Input: part model. Units: mm. Frame: model coordinates. Round coordinates to 2 decimals unless told otherwise and drop trailing zeros. Order: outer loops, then holes, each group sorted by start corner. A loop starts at its lowest first (then second) coordinate and runs counter-clockwise, first axis right, second up. Notation, with made-up numbers: (83.25, -27) -> (97.25, -27) arc R24 cw to (97.25, 4) -> close; hole circle Ø3 at (29.25, -19.5). An arc over 180 degrees is marked (long way). Use a Markdown table: item, result.
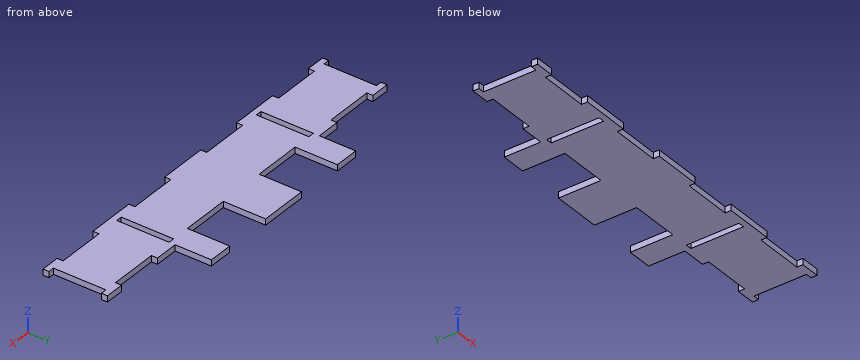
from build123d import *

# Parameters (mm, degrees)
SKETCH1_W           = 395.4
SKETCH1_H           = 67.700000012
BOSS_EXTRUDE1_DEPTH = 6.35
SKETCH2_W           = 50.8
SKETCH2_H           = 6.35
SKETCH2_W_2         = 6.35
SKETCH2_H_2         = 55.000000012
CUT_EXTRUDE1_DEPTH  = 201.677440188
SKETCH5_W           = 6.35
SKETCH5_H           = 55.000000012
CUT_EXTRUDE2_DEPTH  = 201.677440188
SKETCH6_W           = 25.8625
SKETCH6_H           = 6.35
SKETCH6_W_2         = 50.8
BOSS_EXTRUDE2_DEPTH = 38.1


with BuildPart() as part:
    # Sketch1 → Boss-Extrude1 (new body)
    with BuildSketch(Plane.XY):
        Rectangle(SKETCH1_W, SKETCH1_H)
    extrude(amount=BOSS_EXTRUDE1_DEPTH)

    # Sketch2 → Cut-Extrude1 (cut, through all)
    with BuildSketch(Plane.XY.offset(6.35)):
        with Locations((-152.4, -30.675000006)):
            Rectangle(SKETCH2_W, SKETCH2_H)
        with Locations((-152.4, 30.675000006)):
            Rectangle(SKETCH2_W, SKETCH2_H)
        with Locations((-50.8, 30.675000006)):
            Rectangle(SKETCH2_W, SKETCH2_H)
        with Locations((-50.8, -30.675000006)):
            Rectangle(SKETCH2_W, SKETCH2_H)
        with Locations((50.8, -30.675000006)):
            Rectangle(SKETCH2_W, SKETCH2_H)
        with Locations((50.8, 30.675000006)):
            Rectangle(SKETCH2_W, SKETCH2_H)
        with Locations((152.4, 30.675000006)):
            Rectangle(SKETCH2_W, SKETCH2_H)
        with Locations((152.4, -30.675000006)):
            Rectangle(SKETCH2_W, SKETCH2_H)
        with Locations((-98.8875, 0)):
            Rectangle(SKETCH2_W_2, SKETCH2_H_2)
        with Locations((98.8875, 0)):
            Rectangle(SKETCH2_W_2, SKETCH2_H_2)
    extrude(amount=-CUT_EXTRUDE1_DEPTH, mode=Mode.SUBTRACT)

    # Sketch5 → Cut-Extrude2 (cut, through all)
    with BuildSketch(Plane.XY.offset(6.35)):
        with Locations((-194.525, 0)):
            Rectangle(SKETCH5_W, SKETCH5_H)
        with Locations((194.525, 0)):
            Rectangle(SKETCH5_W, SKETCH5_H)
    extrude(amount=-CUT_EXTRUDE2_DEPTH, mode=Mode.SUBTRACT)

    # Sketch6 → Boss-Extrude2 (add)
    with BuildSketch(Plane(origin=(0, 33.850000006, 0), x_dir=(1, 0, 0), z_dir=(0, 1, 0))):
        with Locations((89.13125, -3.175)):
            Rectangle(SKETCH6_W, SKETCH6_H)
        with Locations((0, -3.175)):
            Rectangle(SKETCH6_W_2, SKETCH6_H)
        with Locations((-89.13125, -3.175)):
            Rectangle(SKETCH6_W, SKETCH6_H)
    extrude(amount=BOSS_EXTRUDE2_DEPTH)


solid = part.part
1) Cut plane B-B on z = 2.5. Count the separate pieces of the cut face and the enclosed holes in it, and give its area (3 significant figures).
Results found:
| item | result |
|---|---|
| separate pieces | 1 |
| enclosed holes | 2 |
| area | 26,700 mm² |
2) Pin query (flat end, axial travel): pin 1 Ø1.5 at (y, z) = (-22.5, 1) entering from +X; pin 2 Ø1.9 at (x, z) = (-63, 4) entering from -Y; pin 3 Ø3 at (x, z) = (-154, 4.5) entering from +Y. Return the tip coordinate at first contact, or that it passes through.
Results found:
| item | result |
|---|---|
| pin 1 | stops at x = 191.35 |
| pin 2 | stops at y = -27.5 |
| pin 3 | stops at y = 27.5 |
3) Line query: L1, parallel to X at y = -22, z = 2.5; L2, parallel to X at y = 56.5, z = 3.25; L3, parallel to X at y = -29, z = 3.5. Output: solid intervals per line, ascending. Write a range as [from, to].
Results found:
| item | result |
|---|---|
| L1 | x = [-191.35, -102.06], [-95.71, 95.71], [102.06, 191.35] |
| L2 | x = [-102.06, -76.2], [-25.4, 25.4], [76.2, 102.06] |
| L3 | x = [-197.7, -177.8], [-127, -76.2], [-25.4, 25.4], [76.2, 127], [177.8, 197.7] |
4) Cut plane C-C on x = -52. Return loops of the section in (y, z), and give its area (3 significant figures).
Results found:
| item | result |
|---|---|
| outline | (-27.5, 0) -> (27.5, 0) -> (27.5, 6.35) -> (-27.5, 6.35) -> close |
| area | 349 mm² |
5) Cut plane D-D on y = 11.5. Return loops of the section in (x, z).
Results found:
| item | result |
|---|---|
| outline | (-191.35, 0) -> (-102.06, 0) -> (-102.06, 6.35) -> (-191.35, 6.35) -> close; (-95.71, 0) -> (95.71, 0) -> (95.71, 6.35) -> (-95.71, 6.35) -> close; (102.06, 0) -> (191.35, 0) -> (191.35, 6.35) -> (102.06, 6.35) -> close |
6) Cut plane A-A on y = 52. Return loops of the section in (x, z), and give its area (3 significant figures).
Results found:
| item | result |
|---|---|
| outline | (-102.06, 0) -> (-76.2, 0) -> (-76.2, 6.35) -> (-102.06, 6.35) -> close; (-25.4, 0) -> (25.4, 0) -> (25.4, 6.35) -> (-25.4, 6.35) -> close; (76.2, 0) -> (102.06, 0) -> (102.06, 6.35) -> (76.2, 6.35) -> close |
| area | 651 mm² |
